from build123d import *

# Parameters (mm, degrees)
SKETCH1_W                       = 50.8
SKETCH1_H                       = 50.8
SKETCH1_R                       = 14.2875
BOSS_EXTRUDE1_DEPTH             = 3.175
F_29_0_136_DIAMETER_HOLE1_D     = 3.4544
F_29_0_136_DIAMETER_HOLE1_DEPTH = 38.1
F_29_0_136_DIAMETER_HOLE1_TIP   = 1.037806461


with BuildPart() as part:
    # Sketch1 → Boss-Extrude1 (new, symmetric)
    with BuildSketch(Plane(origin=(0, 0, 0), x_dir=(0, 0, -1), z_dir=(1, 0, 0))):
        Rectangle(SKETCH1_W, SKETCH1_H)
        Circle(SKETCH1_R, mode=Mode.SUBTRACT)
    extrude(amount=BOSS_EXTRUDE1_DEPTH, both=True)

    # #29 (0.136) Diameter Hole1
    with Locations(Plane(origin=(0, 25.4, 20.0025), x_dir=(0, 0, 1), z_dir=(0, 1, 0))):
        with Locations((0, 0), (-40.005, 0)):
            Hole(F_29_0_136_DIAMETER_HOLE1_D / 2, depth=F_29_0_136_DIAMETER_HOLE1_DEPTH)
            with Locations((0, 0, -(F_29_0_136_DIAMETER_HOLE1_DEPTH + F_29_0_136_DIAMETER_HOLE1_TIP / 2))):  # 118° drill point
                Cone(0, F_29_0_136_DIAMETER_HOLE1_D / 2, F_29_0_136_DIAMETER_HOLE1_TIP, mode=Mode.SUBTRACT)


solid = part.part
Check sheet for the modelled part. Datum: model origin and axes. Units: mm. A direction names the side the tool comes from. Round coordinates to 2 decimals unless told otherwise and drop trailing zeros. Order: outer loops, then holes, each group sorted by start corner. A loop starts at its lowest first (then second) coordinate and runs counter-clockwise, first axis right, second up.
(1) Cross-section at A-A, the plane y = 0. Enter the section's corners in (x, z) (1 decimal), and give its area (3 significant figures).
(2) Draft check along X on faces 1 (the flat face through (-3.175, -11, -11)), 2 (the flat face through (3.175, -11, -11)), 3 (the flat face through (0, 25.4, 0)), 4 (the cylindrical face through (0.076, 6.083, -18.277)). Enter one of: pulls with the +X half, pulls with the -X half, needs draft (parallel to the pull), parting line crosses it, or undercut.
(3) Cross-section at D-D, the plane y = -5.5. Enter the section's corners in (x, z) (1 decimal), and give its area (3 significant figures).
(4) Access from +Z, -Z, +X, -X, +Y, -Y to the whole of each face (thin tool, end or side, straight path). Record for faces 5 (the flat face through (0, 0, -25.4)), 6 (the cylindrical face through (0.076, 6.083, 21.728)).
(5) Cross-section at B-B, the plane z = 0. Enter the section's corners in (x, y) (1 decimal).
(6) Go/stop test with a flat-tipped pin: P1, Ø17, axis at y = 0, z = 0, coming from the -X side. Record where the tip stops, or that it passes through.
(7) Scan lines: probe 1 along Z at (x, y) = (0, 16); probe 2 along Z at (x, y) = (1.5, 14.5); probe 3 along Z at (x, y) = (0, 7). Record each from-to range of solid material in increasing order.
(8) Cross-section at C-C, the plane z = 10. Enter the section's corners in (x, y) (3 decimals), and give its area (3 significant figures).
Check sheet entries:
1. outline: (-3.2, -25.4) - (3.2, -25.4) - (3.2, -14.3) - (-3.2, -14.3) - close; (-3.2, 14.3) - (3.2, 14.3) - (3.2, 25.4) - (-3.2, 25.4) - close; hole circle Ø3.5 at (0, -20); hole circle Ø3.5 at (0, 20)
1. area: 122 mm2
2. face 1: pulls with the -X half
2. face 2: pulls with the +X half
2. face 3: needs draft
2. face 4: undercut
3. outline: (-3.2, -25.4) - (3.2, -25.4) - (3.2, -13.2) - (-3.2, -13.2) - close; (-3.2, 13.2) - (3.2, 13.2) - (3.2, 25.4) - (-3.2, 25.4) - close; hole circle Ø3.5 at (0, -20); hole circle Ø3.5 at (0, 20)
3. area: 136 mm2
4. face 5: -Z, +X, -X, +Y, -Y
4. face 6: +Y
5. outline: (-3.2, -25.4) - (3.2, -25.4) - (3.2, -14.3) - (-3.2, -14.3) - close; (-3.2, 14.3) - (3.2, 14.3) - (3.2, 25.4) - (-3.2, 25.4) - close
6. P1: passes through
7. probe 1: z = -25.4 to -21.73, -18.28 to 18.28, 21.73 to 25.4
7. probe 2: z = -25.4 to -20.86, -19.15 to 19.15, 20.86 to 25.4
7. probe 3: z = -25.4 to -21.73, -18.28 to -12.46, 12.46 to 18.28, 21.73 to 25.4
8. outline: (-3.175, -25.4) - (3.175, -25.4) - (3.175, -10.205) - (-3.175, -10.205) - close; (-3.175, 10.205) - (3.175, 10.205) - (3.175, 25.4) - (-3.175, 25.4) - close
8. area: 193 mm2
